Read the model definition and answer for the solid it produces. Units are mm, in the model's axes. Round coordinates to 2 decimals unless told otherwise and drop trailing zeros. Order: outer loops, then holes, each group sorted by start corner. A loop starts at its lowest first (then second) coordinate and runs counter-clockwise, first axis right, second up. Notation, with made-up numbers: (-33, 15) -> (-15, 15) arc R15 ccw to (-15, 40) -> close; hole circle Ø8 at (47, 86.5). An arc over 180 degrees is marked (long way). Use a Markdown table: item, result. Add a question column.
1. Section A-A, the plane y = 3.5 is taken. Give the vertices of the cut face in (x, z), then the cut area to 3 significant figures.
2. Section C-C, the plane x = 3 is taken. Give the vertices of the cut face in (y, z).
3. Section B-B, the plane z = 35 is taken. Give the vertices of the cut face in (x, y).
4. Consider L1, parallel to X at y = -4.25, z = 186; L2, parallel to X at y = 0.5, z = -188; L3, parallel to Y at x = 5.25, z = 141.5. Determine where each line is inside the solid, lowest interval first. Write a range as [from, to].
5. Given pin 1 (5 mm diameter, centred on x = 4, z = -116.5, fed in from -Y); pin 2 (3 mm diameter, centred on x = 3.5, z = -117, fed in from -Y); pin 3 (6 mm diameter, centred on y = 1, z = 61, fed in from +X), each flat-ended and moving along its own axis, determine where each tip first touches the part or whether it passes through.
```python
from build123d import *

# Parameters (mm, degrees)
EXTRUDE_THIN1_DEPTH = 230


with BuildPart() as part:
    # Sketch1 → Extrude-Thin1 (new, symmetric)
    with BuildSketch(Plane.XY):
        Polygon((0, -7.071067812), (7.071067812, 0), (0, 7.071067812), (-7.071067812, 0), align=None)
        Polygon((0, -5.656854249), (5.656854249, 0), (0, 5.656854249), (-5.656854249, 0), align=None, mode=Mode.SUBTRACT)
    extrude(amount=EXTRUDE_THIN1_DEPTH, both=True)


solid = part.part
```
Verdict:
| question | item | result |
|---|---|---|
| 1 | outline | (-3.57, -230) -> (-2.16, -230) -> (-2.16, 230) -> (-3.57, 230) -> close; (2.16, -230) -> (3.57, -230) -> (3.57, 230) -> (2.16, 230) -> close |
| 1 | area | 1,300 mm2 |
| 2 | outline | (-4.07, -230) -> (-2.66, -230) -> (-2.66, 230) -> (-4.07, 230) -> close; (2.66, -230) -> (4.07, -230) -> (4.07, 230) -> (2.66, 230) -> close |
| 3 | outline | (-7.07, 0) -> (0, -7.07) -> (7.07, 0) -> (0, 7.07) -> close; hole (-5.66, 0) -> (0, -5.66) -> (5.66, 0) -> (0, 5.66) -> close |
| 4 | L1 | x = [-2.82, -1.41], [1.41, 2.82] |
| 4 | L2 | x = [-6.57, -5.16], [5.16, 6.57] |
| 4 | L3 | y = [-1.82, -0.41], [0.41, 1.82] |
| 5 | pin 1 | stops at y = -5.57 |
| 5 | pin 2 | stops at y = -5.07 |
| 5 | pin 3 | stops at x = 7.07 |
